The listing builds one solid part. Answer for the finished solid, in the listing's coordinates (mm). Give positions to 0.01 mm unless a question says otherwise; leave off trailing zeros. Order: outer loops, then holes, each group sorted by start corner. A loop starts at its lowest first (then second) coordinate and runs counter-clockwise, first axis right, second up. Notation, with made-up numbers: (51, 51) - (76, 51) arc R22 cw to (76, 76) - close; hole circle Ø1 at (-7, 18). An arc over 180 degrees is marked (long way). Use a Markdown table: item, result. Add a question column.
1) Find section B-B, the plane z = 49.75. Determine the outline of the cut face in (x, y), plus the area to 4 significant figures.
2) Find section A-A, the plane x = 57.25. Determine the outline of the cut face in (y, z).
3) The mould has two halves that part along X. Classify faces 1 (the face through (58.867, -0.493, 49.08)), 2 (the face through (46.674, -0.493, -27.344)), 3 (the face through (-29, 0, 1)): released by +X, released by -X, zero draft, split by the parting line, or undercut.
4) Find section C-C, the plane y = -0.25. State how many separate pieces and enclosed holes the cut face has, plus the area to 3 significant figures.
5) Straight lines are drawn through the part: line 1 (Z direction, x = 13, y = -0.25); line 2 (X direction, y = -0.65, z = 7.5); line 3 (Z direction, x = 57.25, y = -0.4). For each, find the intervals that lie inside material, in ascending order.
from build123d import *

# Parameters (mm, degrees)
F0_R     = 2.778
F0_R_2   = 1.75
F0_R_3   = 1.2
F0_R_4   = 4.1
F0_R_5   = 40
F1_DEPTH = 1


# Not quite as in the source:
# - a feature names something its author has since deleted; it is built from what else it names


with BuildPart() as f1:
    # F0 (on Front) → F1 (new body)
    with BuildSketch(Plane.XZ):
        with BuildLine():
            Line((-62.5, 28.1318609125), (-62.5, -55))
            Line((-62.5, -55), (62.5, -55))
            Line((62.5, -55), (62.5, 55))
            Line((62.5, 55), (-62.5, 55))
            Line((-62.5, 55), (-62.5, 35.8681390875))
            ThreePointArc((-62.5, 35.8681390875), (-58.0625349165, 35.8465893984), (-55.85, 32))
            ThreePointArc((-55.85, 32), (-58.0625349165, 28.1534106016), (-62.5, 28.1318609125))
        make_face()
        with Locations((-25.722, -29.222)):
            Circle(F0_R, mode=Mode.SUBTRACT)
        with Locations((53.25, -40.25)):
            Circle(F0_R_2, mode=Mode.SUBTRACT)
        with Locations((48.722, -29.222)):
            Circle(F0_R, mode=Mode.SUBTRACT)
        with Locations((-60.3, 21.7)):
            Circle(F0_R_3, mode=Mode.SUBTRACT)
        with Locations((-49.6, 25.1)):
            Circle(F0_R_4, mode=Mode.SUBTRACT)
        with Locations((-60.3, 42.3)):
            Circle(F0_R_3, mode=Mode.SUBTRACT)
        with Locations((-25.722, 45.222)):
            Circle(F0_R, mode=Mode.SUBTRACT)
        with Locations((11.5, 8)):
            Circle(F0_R_5, mode=Mode.SUBTRACT)
        with Locations((48.722, 45.222)):
            Circle(F0_R, mode=Mode.SUBTRACT)
        with Locations((57.25, 49.75)):
            Circle(F0_R_2, mode=Mode.SUBTRACT)
    extrude(amount=F1_DEPTH)


solid = f1.part
The answers:
| question | item | result |
|---|---|---|
| 1 | outline | (-62.5, -1) - (55.5, -1) - (55.5, 0) - (-62.5, 0) - close; (59, -1) - (62.5, -1) - (62.5, 0) - (59, 0) - close |
| 1 | area | 121.5 mm2 |
| 2 | outline | (-1, -55) - (0, -55) - (0, 48) - (-1, 48) - close; (-1, 51.5) - (0, 51.5) - (0, 55) - (-1, 55) - close |
| 3 | face 1 | undercut |
| 3 | face 2 | undercut |
| 3 | face 3 | zero draft |
| 4 | separate pieces | 1 |
| 4 | enclosed holes | 10 |
| 4 | area | 8,500 mm2 |
| 5 | line 1 | -55 to -31.97, 47.97 to 55 |
| 5 | line 2 | -62.5 to -28.5, 51.5 to 62.5 |
| 5 | line 3 | -55 to 48, 51.5 to 55 |
